Could you check a few things on this model? Use its own coordinates, in mm. Face numbers are marked on the shaded views. Round coordinates to 2 decimals unless told otherwise and drop trailing zeros. Order: outer loops, then holes, each group sorted by start corner. A loop starts at its lowest first (then second) coordinate and runs counter-clockwise, first axis right, second up. Notation, with made-up numbers: (48, -8.75) - (84, -8.75) arc R19 ccw to (84, 16.25) - close; hole circle Ø7 at (-28, 38). An arc over 180 degrees is marked (long way). Return JSON: item names as keys, results as strings. Group by question number.
from build123d import *

# Parameters (mm, degrees)
SKETCH1_W           = 100
SKETCH1_H           = 53
BOSS_EXTRUDE1_DEPTH = 5
SKETCH2_R           = 1.5875
CUT_EXTRUDE1_DEPTH  = 57.808890149
SKETCH3_W           = 124.759549129
SKETCH3_H           = 83.141448462
BOSS_EXTRUDE2_DEPTH = 9
SKETCH4_W           = 124.759549129
SKETCH4_H           = 83.141448462
BOSS_EXTRUDE3_DEPTH = 5


with BuildPart() as part:
    # Sketch1 → Boss-Extrude1 (new body)
    with BuildSketch(Plane(origin=(0, 0, 0), x_dir=(1, 0, 0), z_dir=(0, 1, 0))):
        Rectangle(SKETCH1_W, SKETCH1_H)
    extrude(amount=BOSS_EXTRUDE1_DEPTH)

    # Sketch2 → Cut-Extrude1 (cut, through all)
    with BuildSketch(Plane.XZ):
        with Locations(Location((46.52, 24.173, 0), (0, 0, 270))):
            Circle(SKETCH2_R)
        with Locations(Location((40.17, -24.087, 0), (0, 0, 270))):
            Circle(SKETCH2_R)
        with Locations(Location((-34.76, -24.087, 0), (0, 0, 270))):
            Circle(SKETCH2_R)
        with Locations(Location((-36.03, 24.173, 0), (0, 0, 270))):
            Circle(SKETCH2_R)
    extrude(amount=-CUT_EXTRUDE1_DEPTH, mode=Mode.SUBTRACT)

    # Sketch3 → Boss-Extrude2 (add)
    with BuildSketch(Plane.XZ):
        with Locations((5.40179994, 9.020492383)):
            Rectangle(SKETCH3_W, SKETCH3_H)
        Polygon((52.6, -11.939816527), (50.354869769, -14.184946758), (50.354869769, -24.628213562), (50, -24.983083332), (50, -26.5), (48.483083332, -26.5), (47.483083332, -27.5), (-51, -27.5), (-51, 27.713), (48.839213562, 27.713), (52.6, 23.952213562), align=None, mode=Mode.SUBTRACT)
    extrude(amount=-BOSS_EXTRUDE2_DEPTH)

    # Sketch4 → Boss-Extrude3 (add)
    with BuildSketch(Plane.XZ):
        with Locations((5.40179994, 9.020492383)):
            Rectangle(SKETCH4_W, SKETCH4_H)
    extrude(amount=-BOSS_EXTRUDE3_DEPTH)


solid = part.part
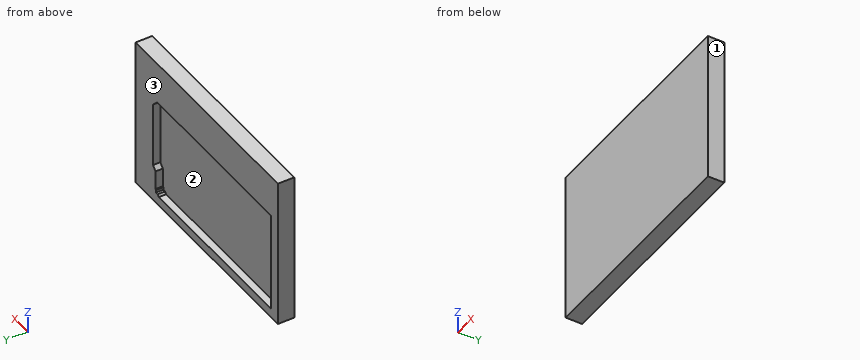
1) We'd pull the mould along X, two halves only. Please class the marked faces 1, 2 and 3: +X half, -X half, draft (parallel to the pull), parting line (faces both ways), or undercut.
2) I want a section at B-B, the plane x = -39.5. List the corners of the cut face in (y, z) for me, plus the area to 3 significant figures.
3) I want a section at A-A, the plane z = 12. List the corners of the cut face in (x, y) for me, plus the area to 3 significant figures.
4) If I drill on line 1 along X through (y, z) = (7.5, 4.5); line 2 along X through (y, z) = (6, -23); line 3 along Z through (x, y) = (5, 5.25), over which ranges is the centre line in solid material (lowest first)? Write a range as from..to.
Outcome:
{
 "1": {"face 1": "+X half", "face 2": "undercut", "face 3": "draft"},
 "2": {"outline": "(0, -32.55) - (9, -32.55) - (9, -27.5) - (5, -27.5) - (5, 27.71) - (9, 27.71) - (9, 50.59) - (0, 50.59) - close", "area": "527 mm^2"},
 "3": {"outline": "(-56.98, 0) - (67.78, 0) - (67.78, 9) - (52.6, 9) - (52.6, 5) - (-51, 5) - (-51, 9) - (-56.98, 9) - close", "area": "708 mm^2"},
 "4": {"line 1": "-56.98..-51, 52.6..67.78", "line 2": "-56.98..-51, 50.35..67.78", "line 3": "-32.55..-27.5, 27.71..50.59"}
}
